For this review, take the finished solid that the model builds, in its own axes (mm). A direction names the side the tool comes from. Round coordinates to 2 decimals unless told otherwise and drop trailing zeros. Write each loop counter-clockwise with the first axis right and the second up, starting at its lowest first coordinate (ties: lowest second). Pieces come first, ordered by that corner, then holes. Notation, with made-up numbers: M 78.25,-33.5 L 97.25,-33.5 A7 ccw 97.25,-21.5 Z; hole C -12.5,-2 d3. An arc over 180 degrees is marked long. Use one line per item in the form item = value. Start each with the question number.
Item 1: For P1, Ø1.1, axis at x = 39, z = -21, coming from the -Y side; P2, Ø0.6, axis at x = 27.5, z = -21, coming from the -Y side; P3, Ø6, axis at x = 15.5, z = -13, coming from the -Y side, all flat-tipped, find the tip position at first contact; note any pin that passes through.
Item 2: For faces 4 (the flat face through (42.45, -1, -21)), 5 (the flat face through (22.49, -2.329, 0.35)), 6 (the cylindrical face through (-0.915, -0.075, -21.299)), list the 3-axis set-ups (+Z, -Z, +X, -X, +Y, -Y) from which the entire face can be reached by the end or side of a thin tool; tool diameter is ignored.
Item 3: Add section C-C (y = 2.5). State the section outline as (x, z) points, and give its area (3 significant figures).
Item 4: Add section A-A (y = -1.5). State the section outline as (x, z) points.
Item 5: Add section B-B (x = 30). State the section outline as (y, z) points, and give its area (3 significant figures).
Item 6: Draft analysis for pull direction Z (two halves, no side actions). For faces 1 (the flat face through (23, -3, 0.7)), 2 (the flat face through (37, 0.1, -21)), 3 (the flat face through (22, 1, -21.6)), state which applies: released by +Z, released by -Z, zero draft, split by the parting line, or undercut.
Item 7: Add section D-D (z = -9). State the section outline as (x, y) points.
Item 8: For line 1 (Z direction, x = 15, y = 1.75); line 2 (X direction, y = 1.25, z = -13.5); line 3 (X direction, y = -2.5, z = -18.25), list the stretches that pass through material, from the lowest coordinate up. Write a range as [from, to].
from build123d import *

# Parameters (mm, degrees)
SKETCH_2_W          = 47.600012207
SKETCH_2_H          = 22.800017408
SKETCH_2_W_2        = 45.600012207
SKETCH_2_H_2        = 20.800017408
EXTRUDE_1_DEPTH     = 1.6
SKETCH_3_W          = 47.600012207
SKETCH_3_H          = 22.800017408
SKETCH_3_W_2        = 45.600012207
SKETCH_3_H_2        = 20.800017408
EXTRUDE_2_DEPTH     = 2
SKETCH_4_W          = 47.600012207
SKETCH_4_H          = 22.800017408
EXTRUDE_3_DEPTH     = 1
SKETCH_5_W          = 47.600012207
SKETCH_5_H          = 22.800017408
SKETCH_5_W_2        = 45.600012207
SKETCH_5_H_2        = 20.800017408
EXTRUDE_4_DEPTH     = 3
SKETCH_6_W          = 8.6
SKETCH_6_H          = 2.628886846
SKETCH_6_W_2        = 13
SKETCH_6_H_2        = 3.428886378
SKETCH_6_W_3        = 10.5
SKETCH_6_H_3        = 3.428887043
CUT_EXTRUDE_1_DEPTH = 1
SKETCH_7_W          = 1.599774972
SKETCH_7_H          = 0.5
SKETCH_7_W_2        = 6.350027001
CUT_EXTRUDE_2_DEPTH = 1
FILLET_1_R          = 1


with BuildPart() as part:
    # Эскиз2 → Бобышка-Вытянуть1 (new body)
    with BuildSketch(Plane(origin=(0, 1.271117687, 0), x_dir=(1, 0, 0), z_dir=(0, 1, 0))):
        with Locations((22.600006104, 10.200008704)):
            Rectangle(SKETCH_2_W, SKETCH_2_H)
        with Locations((22.600006104, 10.200008704)):
            Rectangle(SKETCH_2_W_2, SKETCH_2_H_2, mode=Mode.SUBTRACT)
    extrude(amount=-EXTRUDE_1_DEPTH)

    # Эскиз3 → Бобышка-Вытянуть2 (add)
    with BuildSketch(Plane(origin=(0, 1.271117687, 0), x_dir=(1, 0, 0), z_dir=(0, 1, 0))):
        with Locations((22.600006104, 10.200008704)):
            Rectangle(SKETCH_3_W, SKETCH_3_H)
        with Locations((22.600006104, 10.200008704)):
            Rectangle(SKETCH_3_W_2, SKETCH_3_H_2, mode=Mode.SUBTRACT)
    extrude(amount=EXTRUDE_2_DEPTH)

    # Эскиз4 → Бобышка-Вытянуть3 (add)
    with BuildSketch(Plane(origin=(0, 3.271117687, 0), x_dir=(1, 0, 0), z_dir=(0, 1, 0))):
        with Locations((22.600006104, 10.200008704)):
            Rectangle(SKETCH_4_W, SKETCH_4_H)
    extrude(amount=EXTRUDE_3_DEPTH)

    # Эскиз5 → Бобышка-Вытянуть4 (add)
    with BuildSketch(Plane.XZ.offset(0.328882313)):
        with Locations((22.600006104, -10.200008704)):
            Rectangle(SKETCH_5_W, SKETCH_5_H)
        with Locations((22.600006104, -10.200008704)):
            Rectangle(SKETCH_5_W_2, SKETCH_5_H_2, mode=Mode.SUBTRACT)
    extrude(amount=EXTRUDE_4_DEPTH)

    # Эскиз6 → Вырез-Вытянуть1 (cut)
    with BuildSketch(Plane(origin=(0, 0, -21.600017408), x_dir=(-1, 0, 0), z_dir=(0, 0, -1))):
        with Locations((-21.299859449, -2.01443889)):
            Rectangle(SKETCH_6_W, SKETCH_6_H)
        with Locations((-8.900084477, -1.614439124)):
            Rectangle(SKETCH_6_W_2, SKETCH_6_H_2)
        with Locations((-37.19988645, -1.614438792)):
            Rectangle(SKETCH_6_W_3, SKETCH_6_H_3)
    extrude(amount=-CUT_EXTRUDE_1_DEPTH, mode=Mode.SUBTRACT)

    # Эскиз7 → Вырез-Вытянуть2 (cut)
    with BuildSketch(Plane.XZ.offset(3.328882313)):
        Polygon((-0.2, 0.2), (45.400012207, 0.2), (45.400012207, -20.600017408), (42.44988645, -20.600017408), (42.44988645, -21.100017408), (45.900012207, -21.100017408), (45.900012207, 0.7), (-0.7, 0.7), (-0.7, -21.100017408), (2.400084477, -21.100017408), (2.400084477, -20.600017408), (-0.2, -20.600017408), align=None)
        with Locations((16.199971963, -20.850017408)):
            Rectangle(SKETCH_7_W, SKETCH_7_H)
        with Locations((28.77487295, -20.850017408)):
            Rectangle(SKETCH_7_W_2, SKETCH_7_H)
    extrude(amount=-CUT_EXTRUDE_2_DEPTH, mode=Mode.SUBTRACT)

    # Скругление1
    fillet_1_edges = [part.edges().sort_by_distance(p)[0] for p in [
        (46.400012207, 4.271117687, -10.200008704),
        (22.600006104, 4.271117687, -21.600017408),
        (-1.2, 4.271117687, -10.200008704),
        (22.600006104, 4.271117687, 1.2),
        (-1.2, 0.471117687, 1.2),
        (-1.2, 0.471117687, -21.600017408),
        (46.400012207, 0.471117687, -21.600017408),
        (46.400012207, 0.471117687, 1.2),
    ]]
    fillet(fillet_1_edges, radius=FILLET_1_R)


solid = part.part
Calculated:
q1.P1 = 0.1
q1.P2 = -3.33
q1.P3 = 3.27
q2.face_4 = -Z, -Y
q2.face_5 = -Y
q2.face_6 = -Z, -X, +Y, -Y
q3.outline = M -1.2,-20.6 A1 ccw -0.2,-21.6 L 45.4,-21.6 A1 ccw 46.4,-20.6 L 46.4,0.2 A1 ccw 45.4,1.2 L -0.2,1.2 A1 ccw -1.2,0.2 Z; hole M -0.2,-20.6 L 45.4,-20.6 L 45.4,0.2 L -0.2,0.2 Z
q3.area = 136 mm^2
q4.outline = M -1.2,-20.6 A1 ccw -0.2,-21.6 L 2.4,-21.6 L 2.4,-20.6 L -0.2,-20.6 L -0.2,0.2 L 45.4,0.2 L 45.4,-20.6 L 42.45,-20.6 L 42.45,-21.6 L 45.4,-21.6 A1 ccw 46.4,-20.6 L 46.4,0.2 A1 ccw 45.4,1.2 L -0.2,1.2 A1 ccw -1.2,0.2 Z; M 15.4,-21.6 L 17,-21.6 L 17,-20.6 L 15.4,-20.6 Z; M 25.6,-21.6 L 31.95,-21.6 L 31.95,-20.6 L 25.6,-20.6 Z
q5.outline = M -3.33,-21.6 L 3.27,-21.6 A1 ccw 4.27,-20.6 L 4.27,0.2 A1 ccw 3.27,1.2 L -3.33,1.2 L -3.33,0.7 L -2.33,0.7 L -2.33,0.2 L 3.27,0.2 L 3.27,-20.6 L -2.33,-20.6 L -2.33,-21.1 L -3.33,-21.1 Z
q5.area = 34.6 mm^2
q6.face_1 = undercut
q6.face_2 = zero draft
q6.face_3 = released by -Z
q7.outline = M -1.2,-3.33 L -0.7,-3.33 L -0.7,-2.33 L -0.2,-2.33 L -0.2,3.27 L 45.4,3.27 L 45.4,-2.33 L 45.9,-2.33 L 45.9,-3.33 L 46.4,-3.33 L 46.4,3.27 A1 ccw 45.4,4.27 L -0.2,4.27 A1 ccw -1.2,3.27 Z
q8.line_1 = [-21.6, -20.6], [0.2, 1.2]
q8.line_2 = [-1.2, -0.2], [45.4, 46.4]
q8.line_3 = [-1.2, -0.7], [45.9, 46.4]
